Could you check a few things on this drawing? It's one solid part, dimensions in mm from its lowest x, y, z. A direction names the side the tool comes from. Round coordinates to 2 decimals unless told otherwise and drop trailing zeros. Loops run counter-clockwise (first coordinate to the right, second up) from the corner with the lowest first, then second, coordinate; pieces in that order, holes last. Notation, with made-up numbers: (74, 52) -> (90, 52) arc R26 cw to (90, 73) -> close; hole circle Ø7 at (-30.75, 17.25). An arc over 180 degrees is marked (long way). Use CSV: the item, a comma, the result in double quotes. Start each with the question number.
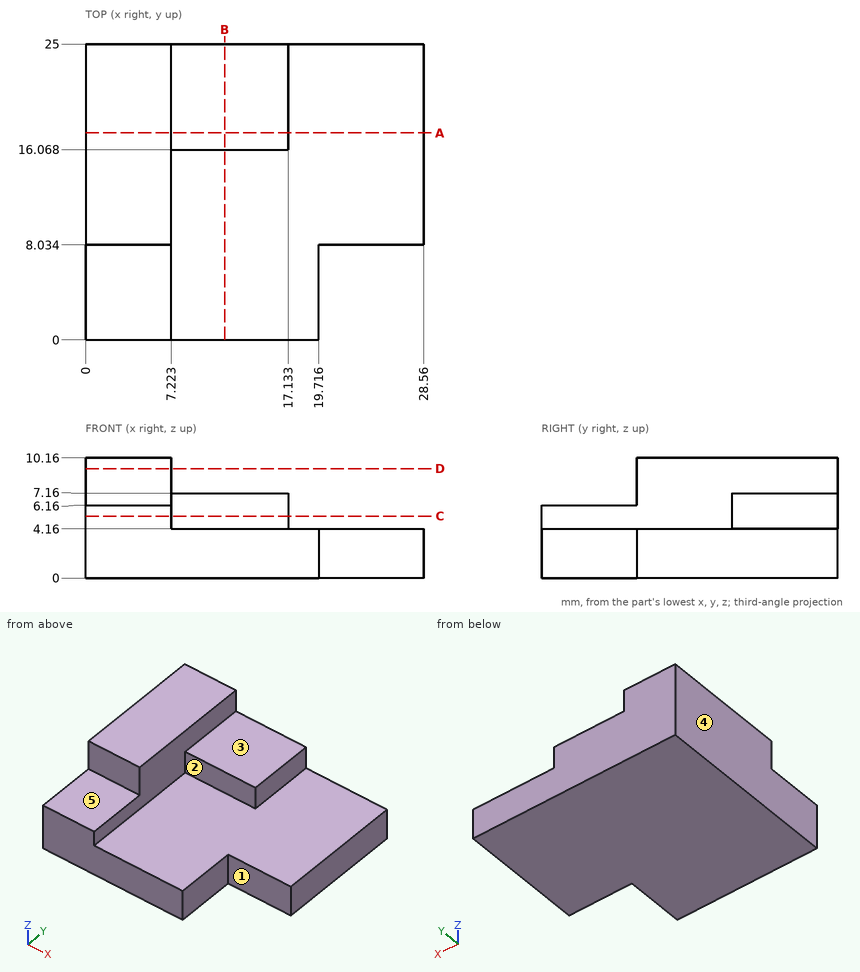
Q1. I want a section at D-D, the plane z = 9.25. List the corners of the cut face in (x, y) for me.
Q2. Will these pins go through, and if not, where does the flat tip stop? pin 1 Ø1.5 at (x, z) = (12.5, 5.5) entering from -Y; pin 2 Ø2 at (x, z) = (6, 1.5) entering from -Y; pin 3 Ø6.5 at (x, y) = (22.5, 15) entering from +Z; pin 4 Ø1 at (y, z) = (9, 5.5) entering from +X.
Q3. I want a section at C-C, the plane z = 5.25. List the corners of the cut face in (x, y) for me, then the cut area to 3 significant figures.
Q4. I want a section at B-B, the plane x = 11.75. List the corners of the cut face in (y, z) for me, then the cut area to 3 significant figures.
Q5. I need wall thicknesses on line 1 along X through (y, z) = (19.25, 7.25); line 2 along Z through (x, y) = (12.25, 15); line 3 along X through (y, z) = (3, 4). Which ranges of each line are inside material? Lowest first, please.
Q6. For the marked faces 1, 2, 3, 4 and 5, which set-ups out of +Z, -Z, +X, -X, +Y, -Y let a thin tool reach every point of the face, with its end or its side?
Q7. I want a section at A-A, the plane y = 17.5. List the corners of the cut face in (x, z) for me.
Values found:
1,outline,"(0, 8.03) -> (7.22, 8.03) -> (7.22, 25) -> (0, 25) -> close"
2,pin 1,"y = 16.07"
2,pin 2,"y = 0"
2,pin 3,"z = 4.16"
2,pin 4,"x = 7.22"
3,outline,"(0, 0) -> (7.22, 0) -> (7.22, 16.07) -> (17.13, 16.07) -> (17.13, 25) -> (0, 25) -> close"
3,area,"269 mm2"
4,outline,"(0, 0) -> (25, 0) -> (25, 7.16) -> (16.07, 7.16) -> (16.07, 4.16) -> (0, 4.16) -> close"
4,area,"131 mm2"
5,line 1,"0 to 7.22"
5,line 2,"0 to 4.16"
5,line 3,"0 to 19.72"
6,face 1,"+Z, -Z, +X, -Y"
6,face 2,"+Z, +X, -Y"
6,face 3,"+Z, +X, +Y, -Y"
6,face 4,"+Z, -Z, -X, +Y, -Y"
6,face 5,"+Z, +X, -X, -Y"
7,outline,"(0, 0) -> (28.56, 0) -> (28.56, 4.16) -> (17.13, 4.16) -> (17.13, 7.16) -> (7.22, 7.16) -> (7.22, 10.16) -> (0, 10.16) -> close"
